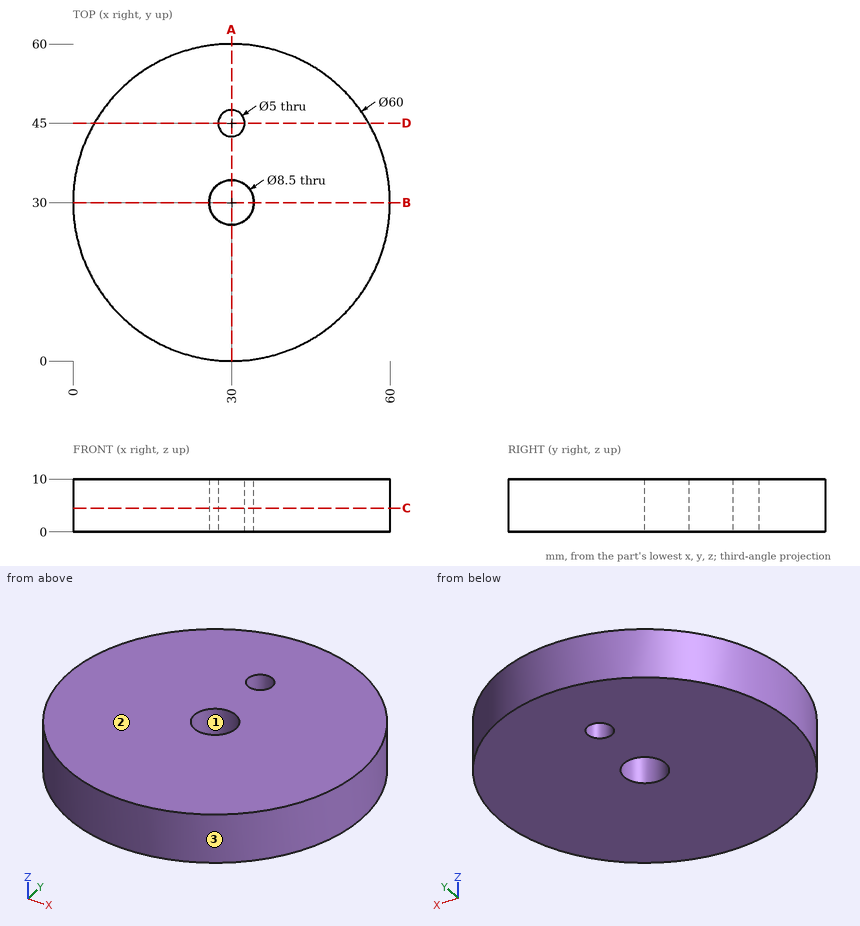
The figure shows three views and two pictorial views of one solid part (mm, origin at its lowest corner). Answer the questions. Coordinates: 2 decimals unless noted, no trailing zeros. Loops run counter-clockwise (first coordinate to the right, second up) from the corner with the lowest first, then second, coordinate; pieces in that order, holes last. Notation, with made-up numbers: M 54,-7 L 84,-7 A14 ccw 84,1 Z; hole C 83.25,51 d7. An arc over 180 degrees is marked long. Answer as CSV lines item,"result". Start each with the question number.
(1) Given pin 1 (5 mm diameter, centred on x = 30, y = 30, fed in from +Z); pin 2 (4 mm diameter, centred on x = 6.5, y = 31.5, fed in from -Z); pin 3 (5 mm diameter, centred on x = 33, z = 6, fed in from -Y); pin 4 (3 mm diameter, centred on x = 53, z = 2.5, fed in from -Y), each flat-ended and moving along its own axis, determine where each tip first touches the part or whether it passes through.
(2) The part is cut by section C-C (z = 4.5). Give the vertices of the cut face in (x, y).
(3) The mould has two halves that part along X. Classify the marked faces 1, 2 and 3: pulls with the +X half, pulls with the -X half, needs draft (parallel to the pull), parting line crosses it, or undercut.
(4) The part is cut by section D-D (y = 45). Give the vertices of the cut face in (x, z), and give its area (3 significant figures).
(5) Find the intervals of material crossed by L1, parallel to Y at x = 30, z = 4.25; L2, parallel to Y at x = 28.5, z = 3.25; L3, parallel to Y at x = 27, z = 9.5, in increasing order. Write a range as [from, to].
(6) The part is cut by section A-A (x = 30). Give the vertices of the cut face in (y, z).
(7) The part is cut by section B-B (y = 30). Give the vertices of the cut face in (x, z).
Determined:
1,pin 1,"through"
1,pin 2,"z = 0"
1,pin 3,"y = 0"
1,pin 4,"y = 9.08"
2,outline,"C 30,30 d60; hole C 30,30 d8.5; hole C 30,45 d5"
3,face 1,"undercut"
3,face 2,"needs draft"
3,face 3,"parting line crosses it"
4,outline,"M 4.02,0 L 27.5,0 L 27.5,10 L 4.02,10 Z; M 32.5,0 L 55.98,0 L 55.98,10 L 32.5,10 Z"
4,area,"470 mm2"
5,L1,"[0, 25.75], [34.25, 42.5], [47.5, 60]"
5,L2,"[0.04, 26.02], [33.98, 43], [47, 59.96]"
5,L3,"[0.15, 26.99], [33.01, 59.85]"
6,outline,"M 0,0 L 25.75,0 L 25.75,10 L 0,10 Z; M 34.25,0 L 42.5,0 L 42.5,10 L 34.25,10 Z; M 47.5,0 L 60,0 L 60,10 L 47.5,10 Z"
7,outline,"M 0,0 L 25.75,0 L 25.75,10 L 0,10 Z; M 34.25,0 L 60,0 L 60,10 L 34.25,10 Z"
